from build123d import *

# Parameters (mm, degrees)
SKETCH1_W           = 63
SKETCH1_H           = 58.5
BOSS_EXTRUDE1_DEPTH = 15
SKETCH2_W           = 84.5
SKETCH2_H           = 56.4
BOSS_EXTRUDE2_DEPTH = 22.5
SKETCH3_W           = 70
SKETCH3_H           = 38
BOSS_EXTRUDE3_DEPTH = 28


with BuildPart() as part:
    # Sketch1 → Boss-Extrude1 (new body)
    with BuildSketch(Plane(origin=(0, 0, 0), x_dir=(1, 0, 0), z_dir=(0, 1, 0))):
        Rectangle(SKETCH1_W, SKETCH1_H)
    extrude(amount=BOSS_EXTRUDE1_DEPTH)

    # Sketch2 → Boss-Extrude2 (add)
    with BuildSketch(Plane(origin=(0, 15, 0), x_dir=(1, 0, 0), z_dir=(0, 1, 0))):
        Rectangle(SKETCH2_W, SKETCH2_H)
    extrude(amount=BOSS_EXTRUDE2_DEPTH)

    # Sketch3 → Boss-Extrude3 (add)
    with BuildSketch(Plane(origin=(0, 37.5, 0), x_dir=(1, 0, 0), z_dir=(0, 1, 0))):
        Rectangle(SKETCH3_W, SKETCH3_H)
    extrude(amount=BOSS_EXTRUDE3_DEPTH)


solid = part.part
Here's how the part is built. I have some questions about the finished solid (model axes, mm). A direction names the side the tool comes from. Coordinates: 2 decimals unless noted, no trailing zeros. Write each loop counter-clockwise with the first axis right and the second up, starting at its lowest first coordinate (ties: lowest second). Pieces come first, ordered by that corner, then holes.
1) If we section it at B-B (z = 21.5): List the corners of the cut face in (x, y) for me.
Filled in:
outline: (-42.25, 15) - (-31.5, 15) - (-31.5, 0) - (31.5, 0) - (31.5, 15) - (42.25, 15) - (42.25, 37.5) - (-42.25, 37.5) - close
2) If we section it at A-A (x = 25.5): List the corners of the cut face in (y, z) for me, plus the area to 3 significant figures.
Filled in:
outline: (0, -29.25) - (15, -29.25) - (15, -28.2) - (37.5, -28.2) - (37.5, -19) - (65.5, -19) - (65.5, 19) - (37.5, 19) - (37.5, 28.2) - (15, 28.2) - (15, 29.25) - (0, 29.25) - close
area: 3,210 mm2
3) If we section it at C-C (y = 48): List the corners of the cut face in (x, z) for me, plus the area to 3 significant figures.
Filled in:
outline: (-35, -19) - (35, -19) - (35, 19) - (-35, 19) - close
area: 2,660 mm2
4) Which directions (+Z, -Z, +X, -X, +Y, -Y) give clear straight access to the entire face, cutting with the end or side of a thin tool? Please do faces 1 (the face through (35, 51, 0)), 2 (the face through (-35, 51, 0)), 3 (the face through (0, 51, -19)), 4 (the face through (-1, 26, 28.2)), 5 (the face through (31.5, 7, 0)).
Filled in:
face 1: +Z, -Z, +X, +Y
face 2: +Z, -Z, -X, +Y
face 3: -Z, +X, -X, +Y
face 4: +Z, +X, -X, +Y
face 5: +Z, -Z, +X, -Y
5) I'm going to push flat-ended pins straight in: pin 1 (12 mm diameter, centred on x = 8, y = 38.5, fed in from -Z); pin 2 (22.5 mm diameter, centred on y = 52, z = 4.5, fed in from -X); pin 3 (5 mm diameter, centred on y = 41, z = -20, fed in from +X). Where does each tip first touch, or does it pass through?
Filled in:
pin 1: stops at z = -28.2
pin 2: stops at x = -35
pin 3: stops at x = 35
6) If I drill on line 1 (X direction, y = 9, z = -9.5); line 2 (Z direction, x = 12, y = 42.5); line 3 (Z direction, x = 14.5, y = 23), over which ranges is the centre line in solid material (lowest first)?
Filled in:
line 1: x = -31.5 to 31.5
line 2: z = -19 to 19
line 3: z = -28.2 to 28.2
7) If we section it at D-D (z = -10): List the corners of the cut face in (x, y) for me, plus the area to 3 significant figures.
Filled in:
outline: (-42.25, 15) - (-31.5, 15) - (-31.5, 0) - (31.5, 0) - (31.5, 15) - (42.25, 15) - (42.25, 37.5) - (35, 37.5) - (35, 65.5) - (-35, 65.5) - (-35, 37.5) - (-42.25, 37.5) - close
area: 4,810 mm2
